CAD build for the part. Positions are in the model's coordinates, mm. A direction names the side the tool comes from. Give positions to 0.01 mm unless a question says otherwise; leave off trailing zeros. Order: outer loops, then holes, each group sorted by start corner. A loop starts at its lowest first (then second) coordinate and runs counter-clockwise, first axis right, second up. Notation, with made-up numbers: (81.5, 57) -> (133.5, 57) arc R19 cw to (133.5, 93) -> close; hole circle Ø5 at (42, -28.5). An arc over 180 degrees is marked (long way). Use one line per item in the form item = value. Start each with the question number.
1) Tool access for faces 5 (the face through (64, 31.75, 29)), 6 (the face through (100, 19, 12.7)), 7 (the face through (98, 38.1, 6)), 8 (the face through (98, 0, 6)), 9 (the face through (29, 38.1, 6)): list every direction of +Z, -Z, +X, -X, +Y, -Y with a clear straight run to the whole face (end or side of a thin tool).
2) Cut at C-C, the plane y = 41.5. Give the cut face in (x, z), and give its area (3 significant figures).
3) Cut at A-A, the plane z = 24. Give the cut face in (x, y).
4) Probe line 1 (X direction, y = 19, z = 6); line 2 (Z direction, x = 60.5, y = 21); line 3 (Z direction, x = 118, y = 11). List the from-to ranges inside material, lowest first.
5) Cut at B-B, the plane x = 16. Give the cut face in (y, z), and give its area (3 significant figures).
6) Mould opens along X. For faces 1 (the face through (5.43, 5.73, 6.44)), 2 (the face through (121.27, 5.43, 6.44)), 3 (the face through (12.766, 20.957, 6.261)), 4 (the face through (64, 19, 19.05)) say: pulls with the +X half, pulls with the -X half, needs draft (parallel to the pull), parting line crosses it, or undercut.
7) Drop flat-ended pins along their axis: P1, Ø10, axis at y = -1, z = 18, coming from the -X side; P2, Ø12, axis at y = 29, z = 22.5, coming from the +X side; P3, Ø19, axis at x = 23.5, y = 11, coming from the +Z side. Give the stop position or say it passes through.
8) Cut at D-D, the plane x = 71. Give the cut face in (y, z), and give its area (3 significant figures).
from build123d import *

# Parameters (mm, degrees)
F0_W      = 127
F0_H      = 38.1
F1_DEPTH  = 12.7
F3_DEPTH  = 50.8
F5_DEPTH  = 12.7
F6_R      = 19.04999
F8_D      = 12.7
F11_D     = 12.7
F12_W     = 25.4
F12_H     = 25.4
F13_DEPTH = 25.4


# Not quite as in the source:
# - a fillet or chamfer is up to 0.001 mm smaller than in the source, because OpenCascade refuses the exact size


with BuildPart() as f1:
    # F0 (on Top) → F1 (new body)
    with BuildSketch(Plane.XY):
        with Locations((63.5, 19.05)):
            Rectangle(F0_W, F0_H)
    extrude(amount=F1_DEPTH)

    # F2 (on face) → F3 (join)
    with BuildSketch(Plane.XZ):
        Polygon((63.5, 12.7), (63.5, 6.35), (85.3080808081, 8.5308080808), (82.7767857143, 12.7), align=None)
        Polygon((85.3080808081, 8.5308080808), (63.5, 6.35), (88.1273764259, 3.8872623574), align=None)
        Polygon((63.5, 6.35), (63.5, 0), (90.4875, 0), (88.1273764259, 3.8872623574), align=None)
        Polygon((38.8726235741, 3.8872623574), (36.5125, 0), (63.5, 0), (63.5, 6.35), align=None)
        Polygon((41.6919191919, 8.5308080808), (38.8726235741, 3.8872623574), (63.5, 6.35), align=None)
        Polygon((63.5, 12.7), (44.2232142857, 12.7), (41.6919191919, 8.5308080808), (63.5, 6.35), align=None)
        Polygon((63.5, 44.45), (44.2232142857, 12.7), (63.5, 12.7), align=None)
        Polygon((63.5, 44.45), (63.5, 12.7), (82.7767857143, 12.7), align=None)
    extrude(amount=-F3_DEPTH)

    # F4 (on face) → F5 (join)
    with BuildSketch(Plane.XZ):
        Polygon((90.4875, 0), (63.5, 44.45), (36.5125, 0), align=None)
    extrude(amount=F5_DEPTH)

    # F6 (radius 19.05 in the source; OpenCascade refuses exactly that, so slightly less here)
    f6_edges = [f1.edges().sort_by_distance(p)[0] for p in [
        (0, 0, 6.35),
        (0, 38.1, 6.35),
        (127, 38.1, 6.35),
        (127, 0, 6.35),
    ]]
    fillet(f6_edges, radius=F6_R)

    # F8 (through all)
    with Locations(Plane.XY.offset(12.7)):
        with Locations((18.8232142857, 19.05)):
            Hole(F8_D / 2)

    # F11 (through all)
    with Locations(Plane.XY.offset(12.7)):
        with Locations((108.1767857143, 19.05)):
            Hole(F11_D / 2)

    # F12 (on offset) → F13 (cut, symmetric)
    with BuildSketch(Plane.YZ.offset(63.5)):
        with Locations((19.05, 31.75)):
            Rectangle(F12_W, F12_H)
    extrude(amount=F13_DEPTH, both=True, mode=Mode.SUBTRACT)


solid = f1.part
Result:
q1.face_5 = +Z, +X, -X
q1.face_6 = +Z, +X, +Y, -Y
q1.face_7 = +Z, +X, +Y
q1.face_8 = +Z, +X, -Y
q1.face_9 = +Z, -X, +Y
q2.outline = (36.51, 0) -> (90.49, 0) -> (63.5, 44.45) -> close
q2.area = 1,200 mm²
q3.outline = (51.08, -12.7) -> (75.92, -12.7) -> (75.92, 6.35) -> (51.08, 6.35) -> close; (51.08, 31.75) -> (75.92, 31.75) -> (75.92, 50.8) -> (51.08, 50.8) -> close
q4.line_1 = 0 to 12.47, 25.17 to 101.83, 114.53 to 127
q4.line_2 = 0 to 19.05
q4.line_3 = 0 to 12.7
q5.outline = (0.25, 0) -> (13.36, 0) -> (13.36, 12.7) -> (0.25, 12.7) -> close; (24.74, 0) -> (37.85, 0) -> (37.85, 12.7) -> (24.74, 12.7) -> close
q5.area = 333 mm²
q6.face_1 = pulls with the -X half
q6.face_2 = pulls with the +X half
q6.face_3 = undercut
q6.face_4 = needs draft
q7.P1 = 44.41
q7.P2 = 80.47
q7.P3 = 12.7
q8.outline = (-12.7, 0) -> (50.8, 0) -> (50.8, 32.1) -> (31.75, 32.1) -> (31.75, 19.05) -> (6.35, 19.05) -> (6.35, 32.1) -> (-12.7, 32.1) -> close
q8.area = 1,710 mm²
